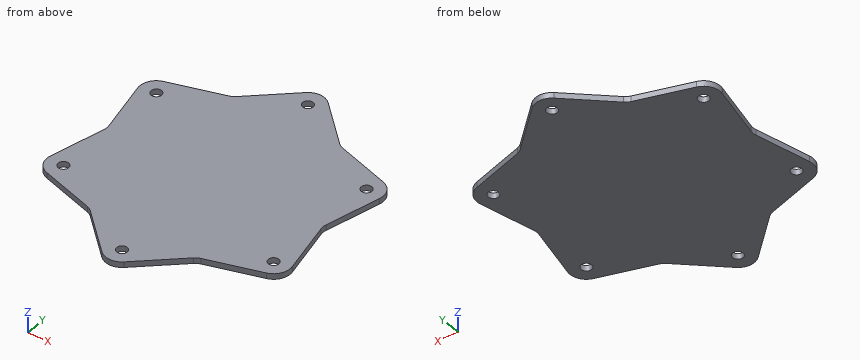
from build123d import *

# Parameters (mm, degrees)
SKETCH1_R           = 3
BOSS_EXTRUDE2_DEPTH = 3.175


with BuildPart() as part:
    # Sketch1 → Boss-Extrude2 (new body)
    with BuildSketch(Plane.XY):
        with BuildLine():
            Line((6.375679422, 76.689094378), (29.728991744, 54.9181954))
            ThreePointArc((29.728991744, 54.9181954), (31.115, 53.892760878), (32.696056474, 53.205159779))
            Line((32.696056474, 53.205159779), (63.226864214, 43.866047535))
            ThreePointArc((63.226864214, 43.866047535), (68.58921198, 39.6), (69.602543635, 32.823046843))
            Line((69.602543635, 32.823046843), (62.425048218, 1.713035621))
            ThreePointArc((62.425048218, 1.713035621), (62.23, 0), (62.425048218, -1.713035621))
            Line((62.425048218, -1.713035621), (69.602543635, -32.823046843))
            ThreePointArc((69.602543635, -32.823046843), (68.58921198, -39.6), (63.226864214, -43.866047535))
            Line((63.226864214, -43.866047535), (32.696056474, -53.205159779))
            ThreePointArc((32.696056474, -53.205159779), (31.115, -53.892760878), (29.728991744, -54.9181954))
            Line((29.728991744, -54.9181954), (6.375679422, -76.689094378))
            ThreePointArc((6.375679422, -76.689094378), (0, -79.2), (-6.375679422, -76.689094378))
            Line((-6.375679422, -76.689094378), (-29.728991744, -54.9181954))
            ThreePointArc((-29.728991744, -54.9181954), (-31.115, -53.892760878), (-32.696056474, -53.205159779))
            Line((-32.696056474, -53.205159779), (-63.226864214, -43.866047535))
            ThreePointArc((-63.226864214, -43.866047535), (-68.58921198, -39.6), (-69.602543635, -32.823046843))
            Line((-69.602543635, -32.823046843), (-62.425048218, -1.713035621))
            ThreePointArc((-62.425048218, -1.713035621), (-62.23, 0), (-62.425048218, 1.713035621))
            Line((-62.425048218, 1.713035621), (-69.602543635, 32.823046843))
            ThreePointArc((-69.602543635, 32.823046843), (-68.58921198, 39.6), (-63.226864214, 43.866047535))
            Line((-63.226864214, 43.866047535), (-32.696056474, 53.205159779))
            ThreePointArc((-32.696056474, 53.205159779), (-31.115, 53.892760878), (-29.728991744, 54.9181954))
            Line((-29.728991744, 54.9181954), (-6.375679422, 76.689094378))
            ThreePointArc((-6.375679422, 76.689094378), (0, 79.2), (6.375679422, 76.689094378))
        make_face()
        with Locations((0, 69.85)):
            Circle(SKETCH1_R, mode=Mode.SUBTRACT)
        with Locations((60.491874454, 34.925)):
            Circle(SKETCH1_R, mode=Mode.SUBTRACT)
        with Locations((60.491874454, -34.925)):
            Circle(SKETCH1_R, mode=Mode.SUBTRACT)
        with Locations((0, -69.85)):
            Circle(SKETCH1_R, mode=Mode.SUBTRACT)
        with Locations((-60.491874454, -34.925)):
            Circle(SKETCH1_R, mode=Mode.SUBTRACT)
        with Locations((-60.491874454, 34.925)):
            Circle(SKETCH1_R, mode=Mode.SUBTRACT)
    extrude(amount=BOSS_EXTRUDE2_DEPTH)


solid = part.part
Can you work these out from the model? Positions are in its coordinate system, mm. Give positions to 0.01 mm unless a question says otherwise; leave off trailing zeros. Order: outer loops, then holes, each group sorted by start corner. A loop starts at its lowest first (then second) coordinate and runs counter-clockwise, first axis right, second up. Notation, with made-up numbers: M 32,79.5 L 63,79.5 A20 ccw 63,101.5 Z; hole C 87,34.25 d5. An arc over 180 degrees is marked long. Use one line per item in the form item = value. Start each with the question number.
Item 1: If we section it at A-A (x = 0): Write out the boundary of the cut face in (y, z) (3 decimals), then the cut area to 3 significant figures.
Item 2: Will these pins go through, and if not, where does the flat tip stop? pin 1 Ø1.5 at (y, z) = (40.5, 2.5) entering from -X; pin 2 Ø5 at (x, y) = (0, -69.85) entering from +Z; pin 3 Ø1.5 at (y, z) = (-2.5, 1) entering from -X.
Item 3: If we section it at C-C (z = 2.2): State how many separate pieces and enclosed holes the cut face has, then the cut area to 3 significant figures.
Item 4: If I drill on line 1 along Y through (x, z) = (0, 2.35); line 2 along Y through (x, z) = (2, 2.15); line 3 along X through (y, z) = (-35, 2.95), over which ranges is the centre line in solid material (lowest first)?
Item 5: If we section it at D-D (x = -43): Write out the boundary of the cut face in (y, z) (3 decimals), then the cut area to 3 significant figures.
Item 6: If we section it at B-B (y = -69.85): Write out the boundary of the cut face in (x, z) (3 decimals), then the cut area to 3 significant figures.
Outcome:
q1.outline = M -79.2,0 L -72.85,0 L -72.85,3.175 L -79.2,3.175 Z; M -66.85,0 L 66.85,0 L 66.85,3.175 L -66.85,3.175 Z; M 72.85,0 L 79.2,0 L 79.2,3.175 L 72.85,3.175 Z
q1.area = 465 mm2
q2.pin_1 = -68.5
q2.pin_2 = through
q2.pin_3 = -62.78
q3.separate_pieces = 1
q3.enclosed_holes = 6
q3.area = 15,100 mm2
q4.line_1 = -79.2 to -72.85, -66.85 to 66.85, 72.85 to 79.2
q4.line_2 = -78.98 to -72.09, -67.61 to 67.61, 72.09 to 78.98
q4.line_3 = -69.84 to -63.49, -57.49 to 57.49, 63.49 to 69.84
q5.outline = M -50.053,0 L 50.053,0 L 50.053,3.175 L -50.053,3.175 Z
q5.area = 318 mm2
q6.outline = M -13.712,0 L -3,0 L -3,3.175 L -13.712,3.175 Z; M 3,0 L 13.712,0 L 13.712,3.175 L 3,3.175 Z
q6.area = 68.0 mm2
